Design review of the part shown in the three views and the two pictorial views. Dimensions are in mm from the part's minimum x, y and z. A direction names the side the tool comes from. Round coordinates to 2 decimals unless told otherwise and drop trailing zeros. Write each loop counter-clockwise with the first axis right and the second up, starting at its lowest first coordinate (ties: lowest second). Pieces come first, ordered by that corner, then holes. Notation, with made-up numbers: (-1.75, 82) - (32.25, 82) arc R15 cw to (32.25, 110) - close; hole circle Ø9 at (15, 5). An arc over 180 degrees is marked (long way). Use one line per item in the form item = value.
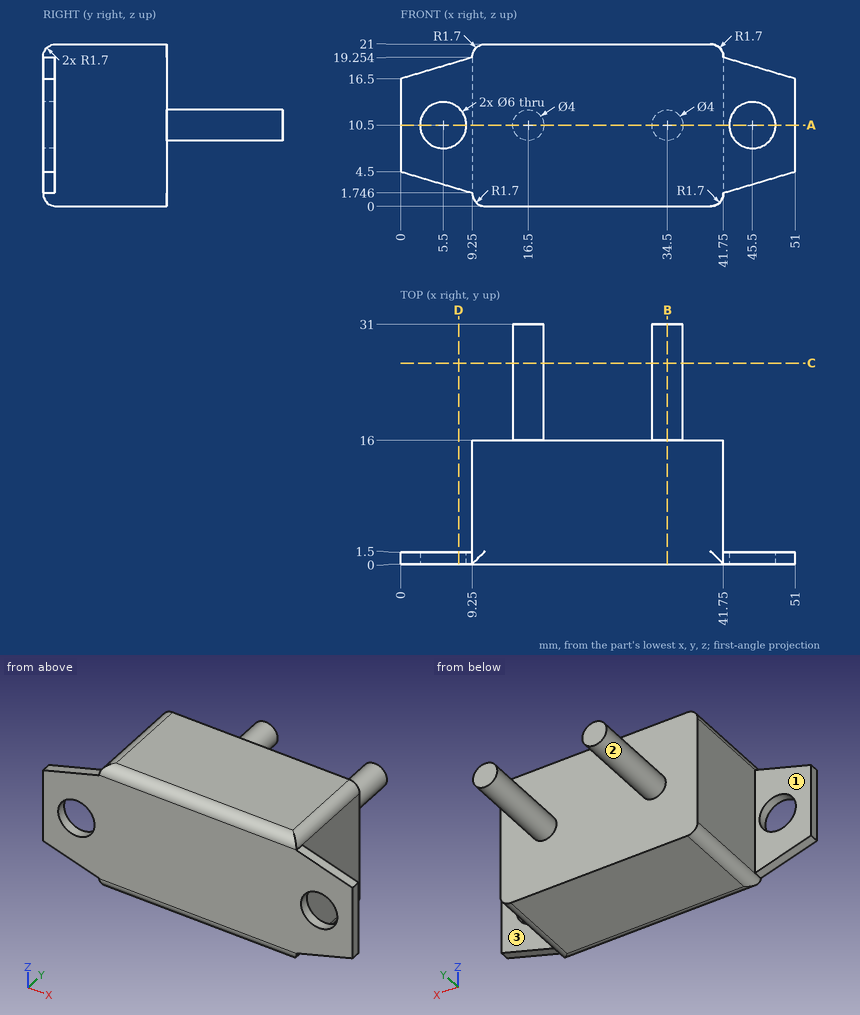
(1) Add section B-B on x = 34.5. Write out the cut boundary in (y, z), then the cut area to 3 significant figures.
Geometry results:
outline = (0, 1.7) arc R1.7 ccw to (1.7, 0) - (16, 0) - (16, 8.5) - (31, 8.5) - (31, 12.5) - (16, 12.5) - (16, 21) - (1.7, 21) arc R1.7 ccw to (0, 19.3) - close
area = 395 mm2
(2) To check wall thickness, follow L1, parallel to Y at x = 20, z = 5; L2, parallel to X at y = 9, z = 1.5; L3, parallel to X at y = 13, z = 14. State the ranges of each line that lie inside material, in increasing order.
Geometry results:
L1 = 0 to 16
L2 = 9.26 to 41.74
L3 = 9.25 to 41.75
(3) Add section D-D on x = 7.5. Write out the cut boundary in (y, z).
Geometry results:
outline = (0, 2.27) - (1.5, 2.27) - (1.5, 8.26) - (0, 8.26) - close; (0, 12.74) - (1.5, 12.74) - (1.5, 18.73) - (0, 18.73) - close
(4) Insertion check: P1, Ø1.5, axis at y = 8.5, z = 11, coming from the +X side; P2, Ø7.5, axis at x = 6.5, z = 8.5, coming from the +Y side; P3, Ø10, axis at x = 47.5, z = 7, coming from the +Y side; P4, Ø8, axis at x = 26, y = 21.5, coming from the -Z side. Each pin has a flat end and moves straight along its axis. Give the tip position at first contact, or say it passes through.
Geometry results:
P1 = 41.75
P2 = 16
P3 = 1.5
P4 = through
(5) Machinability: for the marked faces 1, 2 and 3, which of the approach directions +Z, -Z, +X, -X, +Y, -Y give a long, thin tool a straight path to every point of the face, cutting with its end or side? Answer none if there is none.
Geometry results:
face_1 = +Z, -Z, -X, +Y
face_2 = +Y
face_3 = +Z, -Z, +X, +Y
(6) Add section A-A on z = 10.5. Write out the cut boundary in (x, y), then the cut area to 3 significant figures.
Geometry results:
outline = (0, 0) - (2.5, 0) - (2.5, 1.5) - (0, 1.5) - close; (8.5, 0) - (42.5, 0) - (42.5, 1.5) - (41.75, 1.5) - (41.75, 16) - (36.5, 16) - (36.5, 31) - (32.5, 31) - (32.5, 16) - (18.5, 16) - (18.5, 31) - (14.5, 31) - (14.5, 16) - (9.25, 16) - (9.25, 1.5) - (8.5, 1.5) - close; (48.5, 0) - (51, 0) - (51, 1.5) - (48.5, 1.5) - close
area = 650 mm2
(7) Add section C-C on y = 26. Write out the cut boundary in (x, z).
Geometry results:
outline = circle Ø4 at (16.5, 10.5); circle Ø4 at (34.5, 10.5)
